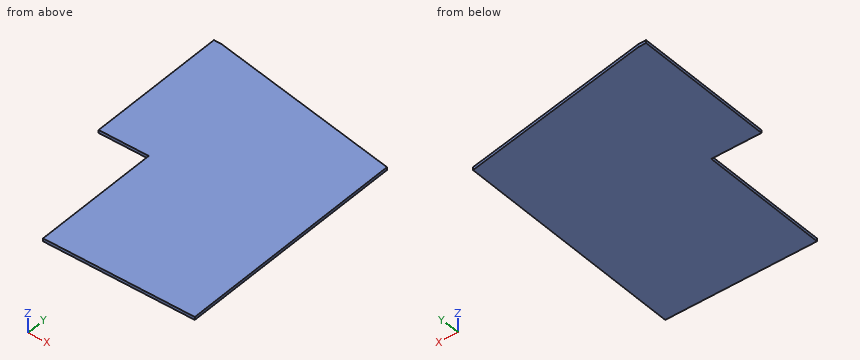
```python
from build123d import *

# Parameters (mm, degrees)
TABAN_FLAN_1_DEPTH         = 10
KES_EKSTR_ZYON1_DEPTH      = 2664.925674639
KES_EKSTR_ZYON1_DEPTH_BACK = 2664.925674639
IZIM2_W                    = 1985
IZIM2_H                    = 440
KES_EKSTR_ZYON2_DEPTH      = 2664.925674639
KES_EKSTR_ZYON2_DEPTH_BACK = 2664.925674639
IZIM4_W                    = 2142.353076874
IZIM4_H                    = 1059.200267334
KES_EKSTR_ZYON3_DEPTH      = 2664.925674639
KES_EKSTR_ZYON3_DEPTH_BACK = 2664.925674639
IZIM5_W                    = 190.659324766
IZIM5_H                    = 598.86582779


# Sheet-metal steps are written as plain solids
with BuildPart() as part:
    # Çizim1 → Taban-Flanş1 (new body)
    with BuildSketch(Plane.XY):
        Polygon((0, 0), (0, 800), (660, 920), (1840, 920), (2500, 800), (2500, 0), align=None)
    extrude(amount=-TABAN_FLAN_1_DEPTH)

    # Çizim2 → Kes-Ekstrüzyon1 (cut, two sides: drawn at the far end of the back side and taken through both)
    with BuildSketch(Plane.XY.offset(-KES_EKSTR_ZYON1_DEPTH_BACK)):
        with Locations((992.5, 220)):
            Rectangle(IZIM2_W, IZIM2_H)
    extrude(amount=KES_EKSTR_ZYON1_DEPTH + KES_EKSTR_ZYON1_DEPTH_BACK, mode=Mode.SUBTRACT)

    # Çizim4 → Kes-Ekstrüzyon2 (cut, two sides: drawn at the far end of the back side and taken through both)
    with BuildSketch(Plane.XY.offset(-KES_EKSTR_ZYON2_DEPTH_BACK)):
        with Locations((741.823461563, 774.473780937)):
            Rectangle(IZIM4_W, IZIM4_H)
    extrude(amount=KES_EKSTR_ZYON2_DEPTH + KES_EKSTR_ZYON2_DEPTH_BACK, mode=Mode.SUBTRACT)

    # Çizim5 → Kes-Ekstrüzyon3 (cut, two sides: drawn at the far end of the back side and taken through both)
    with BuildSketch(Plane.XY.offset(-KES_EKSTR_ZYON3_DEPTH_BACK)):
        with Locations((1719.670337617, 680.404157963)):
            Rectangle(IZIM5_W, IZIM5_H)
    extrude(amount=KES_EKSTR_ZYON3_DEPTH + KES_EKSTR_ZYON3_DEPTH_BACK, mode=Mode.SUBTRACT)


solid = part.part
```
Source: CAD feature listing. Evaluate the final solid. Frame: model axes, mm. Coordinates: 2 decimals unless noted, no trailing zeros. Loops run counter-clockwise (first coordinate to the right, second up) from the corner with the lowest first, then second, coordinate; pieces in that order, holes last. Notation, with made-up numbers: (-35, 43.25) -> (3, 43.25) arc R11 ccw to (3, 59.25) -> close; hole circle Ø2 at (-4.5, 67). An arc over 180 degrees is marked (long way). One line per item, written item: value. Start each with the question number.
Q1. Contact query for flat-ended pins moving along their axis: P1, Ø3, axis at x = 1865, z = -2.5, coming from the -Y side; P2, Ø6, axis at x = 1963.5, z = -6, coming from the +Y side; P3, Ø5, axis at y = 131.5, z = -6.5, coming from the -X side. Output: stop coordinate, or through.
Q2. Section query A-A, the plane z = -3.5. Return the cut outline in (x, y).
Q3. Section query B-B, the plane y = 344. Return the cut outline in (x, z).
Q4. Section query C-C, the plane x = 2173. Return the cut outline in (y, z), and give its area (3 significant figures).
Q5. Line query: line 1 along X through (y, z) = (347, -6.75); line 2 along Y through (x, z) = (2280, -0.5); line 3 along Y through (x, z) = (2317, -0.5). Output: solid intervals per line, ascending.
Results:
1. P1: y = 440
1. P2: y = 898.09
1. P3: x = 1985
2. outline: (1815, 440) -> (1985, 440) -> (1985, 0) -> (2500, 0) -> (2500, 800) -> (1840, 920) -> (1815, 920) -> close
3. outline: (1985, -10) -> (2500, -10) -> (2500, 0) -> (1985, 0) -> close
4. outline: (0, -10) -> (859.45, -10) -> (859.45, 0) -> (0, 0) -> close
4. area: 8,590 mm^2
5. line 1: 1985 to 2500
5. line 2: 0 to 840
5. line 3: 0 to 833.27
